Work out the finished part from the listing and answer in its coordinate system (mm). A direction names the side the tool comes from. Give positions to 0.01 mm unless a question says otherwise; leave off trailing zeros. Write each loop counter-clockwise with the first axis right and the second up, starting at its lowest first coordinate (ties: lowest second). Pieces come first, ordered by that corner, then holes. Notation, with made-up numbers: (89.5, 27) -> (131.5, 27) arc R17 cw to (131.5, 34) -> close; hole circle Ø5 at (22, 67.25). An arc over 180 degrees is marked (long way). Use a Markdown table: item, result. Add a question column.
Q1. For a pull along Z with two mould halves and no side action, classify faces 1 (the face through (-20.77, -1.48, 8.2)), 2 (the face through (-16.5, -1.51, 5.22)), 3 (the face through (15.767, -3.409, 4.782)) as pulls with the +Z half, pulls with the -Z half, needs draft (parallel to the pull), parting line crosses it, or undercut.
Q2. Section B-B, the plane y = -4 is taken. Give the vertices of the cut face in (x, z), plus the area to 3 significant figures.
Q3. Section C-C, the plane z = 1.5 is taken. Give the vertices of the cut face in (x, y), plus the area to 3 significant figures.
Q4. For faces 4 (the face through (20, -3, 4)), 5 (the face through (-20, -3, 4)), 6 (the face through (-16, 0, 5)), determine the directions among +Z, -Z, +X, -X, +Y, -Y from which every point of the face is accessible in a straight line to the end or side of a thin tool.
Q5. Consider line 1 (X direction, y = -1.5, z = 4.85); line 2 (X direction, y = -2.1, z = 4.85); line 3 (X direction, y = -7.5, z = 3.5). Determine where each line is inside the solid, lowest interval first.
Q6. Section D-D, the plane x = -4 is taken. Give the vertices of the cut face in (y, z).
Q7. Each of these flat-tipped pins is pushed along its axis until it touches: pin 1 Ø2.5 at (x, z) = (19.5, 4.5) entering from -Y; pin 2 Ø1.5 at (y, z) = (-6.5, 6.5) entering from +X; pin 3 Ø4 at (y, z) = (-8, 3.5) entering from +X. Where does it stop, or does it pass through?
Q8. Section A-A, the plane z = 5.25 is taken. Give the vertices of the cut face in (x, y).
Autodesk Inventor part; units mm, degrees
ref_plane "YZ Plane" through (0, 0, 0) normal (1, 0, 0) x (0, 1, 0)
ref_plane "XZ Plane" through (0, 0, 0) normal (0, 1, 0) x (-1, 0, 0)
ref_plane "XY Plane" through (0, 0, 0) normal (0, 0, 1) x (1, 0, 0)
sketch "Sketch1" plane through (0, 0, 0) normal (0, 0, 1) x (1, 0, 0)
  line L0 (12.7, 0) -> (22.2, 0)
  line L1 (22.2, 0) -> (22.2, -3)
  line L2 (22.2, -3) -> (12.7, -3)
  line L3 (12.7, -3) -> (12.7, 0)
  circle A0 centre (0, 0) radius 12.7
  circle A1 centre (0, 0) radius 15.7
  line L4 (-15.7, 0) -> (-12.7, 0)
  line L5 (12.7, 0) -> (15.7, 0)
  line L6 (-12.7, 0) -> (-22.2, 0)
  line L7 (-22.2, 0) -> (-22.2, -3)
  line L8 (-22.2, -3) -> (-12.7, -3)
  line L9 (-12.7, -3) -> (-12.7, 0)
  dimension "d0" = 12.7
  dimension "d1" = 3
  dimension "d2" = 3
  dimension "d3" = 6.5
extrude "Extrusion1" add sketch "Sketch1" along normal blind 9.7 contours L0 A1 L2 L3 | L3 L2 A1 L8 L9 A0 | L0 L1 L2 A1 | L9 L8 A1 L4 | A1 L8 L7 L6
sketch "Sketch2" plane through (15.4107, -3, 0) normal (0, -1, 0) x (1, 0, 0)
  line L0 (0, 9.7) -> (0, 0)
  line L1 (0, 4.85) -> (2.75, 4.85)
  circle A0 centre (2.75, 4.85) radius 2.75
  point P0 (-15.4107, 0)
  dimension "d6" = 5.5
hole "Hole1" at (18.1607, -3, 4.85) direction (0, 1, 0) diameter 3.4 end through all
ref_plane "Work Plane1" through (0, -3, 0) normal (1, 0, 0) x (0, 0, -1)
mirror "Mirror1" about plane through (0, -3, 0) normal (1, 0, 0) of "Hole1"
fillet "Fillet1" radius 5 2 edges at (-22.2, -1.5, 9.7) (22.2, -1.5, 9.7)
fillet "Fillet1" radius 2 2 edges at (15.4107, -3, 4.85) (-15.4107, -3, 4.85)
properties part number "bottom_fitting"
Result set:
| question | item | result |
|---|---|---|
| 1 | face 1 | pulls with the +Z half |
| 1 | face 2 | undercut |
| 1 | face 3 | needs draft |
| 2 | outline | (-15.25, 0) -> (-12.05, 0) -> (-12.05, 9.7) -> (-15.25, 9.7) -> close; (12.05, 0) -> (15.25, 0) -> (15.25, 9.7) -> (12.05, 9.7) -> close |
| 2 | area | 62.0 mm2 |
| 3 | outline | (-22.2, -3) -> (-16.98, -3) arc R2 cw to (-15.06, -4.44) arc R15.7 ccw to (15.06, -4.44) arc R2 cw to (16.98, -3) -> (22.2, -3) -> (22.2, 0) -> (12.7, 0) arc R12.7 cw to (-12.7, 0) -> (-22.2, 0) -> close |
| 3 | area | 174 mm2 |
| 4 | face 4 | +Z, -Z, +X, -Y |
| 4 | face 5 | +Z, -Z, -X, -Y |
| 4 | face 6 | +Z, -Z, +X, -X, +Y |
| 5 | line 1 | x = -22.2 to -19.86, -16.46 to -12.61, 12.61 to 16.46, 19.86 to 22.2 |
| 5 | line 2 | x = -22.2 to -19.86, -16.46 to -12.53, 12.53 to 16.46, 19.86 to 22.2 |
| 5 | line 3 | x = -13.79 to -10.25, 10.25 to 13.79 |
| 6 | outline | (-15.18, 0) -> (-12.05, 0) -> (-12.05, 9.7) -> (-15.18, 9.7) -> close |
| 7 | pin 1 | stops at y = -3 |
| 7 | pin 2 | stops at x = 14.61 |
| 7 | pin 3 | stops at x = 14.51 |
| 8 | outline | (-22.17, -3) -> (-19.81, -3) -> (-19.81, 0) -> (-22.17, 0) -> close; (-16.51, -3.06) arc R2 cw to (-15.06, -4.44) arc R15.7 ccw to (15.06, -4.44) arc R2 cw to (16.51, -3.06) -> (16.51, 0) -> (12.7, 0) arc R12.7 cw to (-12.7, 0) -> (-16.51, 0) -> close; (19.81, -3) -> (22.17, -3) -> (22.17, 0) -> (19.81, 0) -> close |
